Study the drawing (mm; zero at the part's minimum x, y, z) and answer. A direction names the side the tool comes from. Give positions to 0.01 mm unless a question says otherwise; leave off trailing zeros. Order: outer loops, then holes, each group sorted by start corner. A loop starts at its lowest first (then second) coordinate and runs counter-clockwise, first axis right, second up.
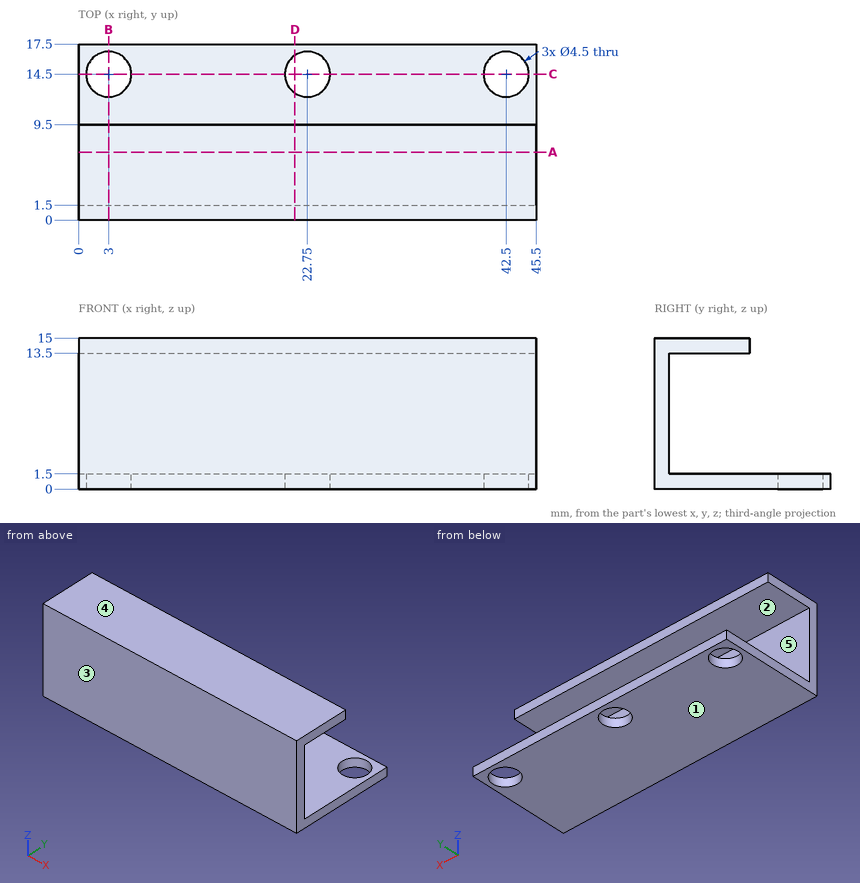
1) Straight lines are drawn through the part: probe 1 along Z at (x, y) = (35, 4); probe 2 along Y at (x, z) = (22.75, 0.85); probe 3 along Z at (x, y) = (33, 11). For each, find the intervals that lie inside material, in ascending order.
Geometry says:
probe 1: z = 0 to 1.5, 13.5 to 15
probe 2: y = 0 to 12.25, 16.75 to 17.5
probe 3: z = 0 to 1.5
2) Given P1, Ø3.5, axis at x = 22.75, y = 14.5, coming from the +Z side; P2, Ø1.6, axis at x = 31, z = 14.5, coming from the +Y side; P3, Ø1.5, axis at x = 16.5, y = 11, coming from the +Z side, each flat-ended and moving along its own axis, determine where each tip first touches the part or whether it passes through.
Geometry says:
P1: passes through
P2: stops at y = 9.5
P3: stops at z = 1.5
3) Find section B-B (x = 3). Write down the section's boundary in (y, z).
Geometry says:
outline: (0, 0) - (12.25, 0) - (12.25, 1.5) - (1.5, 1.5) - (1.5, 13.5) - (9.5, 13.5) - (9.5, 15) - (0, 15) - close; (16.75, 0) - (17.5, 0) - (17.5, 1.5) - (16.75, 1.5) - close
4) Find section C-C (y = 14.5). Write down the section's boundary in (x, z).
Geometry says:
outline: (0, 0) - (0.75, 0) - (0.75, 1.5) - (0, 1.5) - close; (5.25, 0) - (20.5, 0) - (20.5, 1.5) - (5.25, 1.5) - close; (25, 0) - (40.25, 0) - (40.25, 1.5) - (25, 1.5) - close; (44.75, 0) - (45.5, 0) - (45.5, 1.5) - (44.75, 1.5) - close
5) A tool of negligible diameter and unlimited length cuts with its end or side. For the marked faces 4 and 5, from which of +Z, -Z, +X, -X, +Y, -Y can it reach the whole face along a straight path? Write none if from no direction.
Geometry says:
face 4: +Z, +X, -X, +Y, -Y
face 5: +X, -X, +Y
6) Find section D-D (x = 21.5). Write down the section's boundary in (y, z), then the cut area to 3 significant figures.
Geometry says:
outline: (0, 0) - (12.63, 0) - (12.63, 1.5) - (1.5, 1.5) - (1.5, 13.5) - (9.5, 13.5) - (9.5, 15) - (0, 15) - close; (16.37, 0) - (17.5, 0) - (17.5, 1.5) - (16.37, 1.5) - close
area: 52.9 mm2
7) For a pull along Z with two mould halves and no side action, classify the marked faces 1, 2 and 3 as +Z half, -Z half, draft (parallel to the pull), parting line (faces both ways), or undercut.
Geometry says:
face 1: -Z half
face 2: undercut
face 3: draft
8) Find section A-A (y = 6.75). Write down the section's boundary in (x, z), then the cut area to 4 significant figures.
Geometry says:
outline: (0, 0) - (45.5, 0) - (45.5, 1.5) - (0, 1.5) - close; (0, 13.5) - (45.5, 13.5) - (45.5, 15) - (0, 15) - close
area: 136.5 mm2
